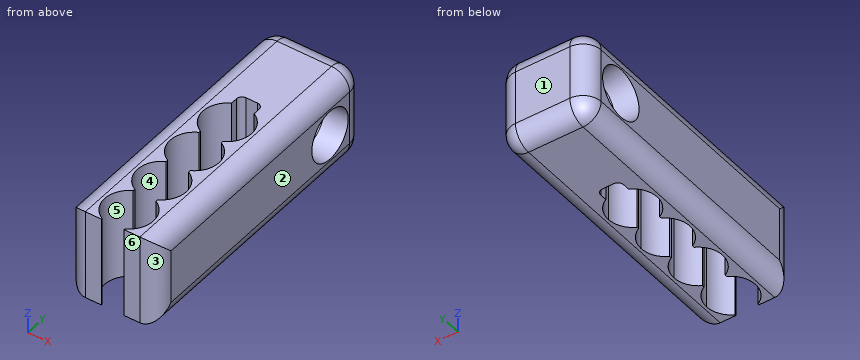
```python
from build123d import *

# Parameters (mm, degrees)
F1_DEPTH = 8
F2_R     = 2.05
F3_DEPTH = 8.001
F4_R     = 1.6
F5_R     = 0.5
F6_SIZE2 = 0.1749773271
F6_SIZE  = 2


with BuildPart() as f1:
    # F0 (on Top) → F1 (new body)
    with BuildSketch(Plane.XY):
        Polygon((1, -4), (4, -4), (4, 4), (-4, 4), (-4, -4), (-1, -4), align=None)
        with BuildLine():
            Line((-1, -5.0967133689), (-1, -4))
            Line((-1, -4), (-4, -4))
            Line((-4, -4), (-4, -21))
            Line((-4, -21), (-1, -21))
            Line((-1, -21), (-1, -20.9032866311))
            ThreePointArc((-1, -20.9032866311), (-2.15, -19), (-1, -17.0967133689))
            Line((-1, -17.0967133689), (-1, -16.9032866311))
            ThreePointArc((-1, -16.9032866311), (-2.15, -15), (-1, -13.0967133689))
            Line((-1, -13.0967133689), (-1, -12.9032866311))
            ThreePointArc((-1, -12.9032866311), (-2.15, -11), (-1, -9.0967133689))
            Line((-1, -9.0967133689), (-1, -8.9032866311))
            ThreePointArc((-1, -8.9032866311), (-2.15, -7), (-1, -5.0967133689))
        make_face()
        with BuildLine():
            Line((4, -21), (4, -4))
            Line((4, -4), (1, -4))
            Line((1, -4), (1, -5.0967133689))
            ThreePointArc((1, -5.0967133689), (1.840176622, -5.8881322021), (2.15, -7))
            ThreePointArc((2.15, -7), (1.840176622, -8.1118677979), (1, -8.9032866311))
            Line((1, -8.9032866311), (1, -9.0967133689))
            ThreePointArc((1, -9.0967133689), (1.840176622, -9.8881322021), (2.15, -11))
            ThreePointArc((2.15, -11), (1.840176622, -12.1118677979), (1, -12.9032866311))
            Line((1, -12.9032866311), (1, -13.0967133689))
            ThreePointArc((1, -13.0967133689), (1.840176622, -13.8881322021), (2.15, -15))
            ThreePointArc((2.15, -15), (1.840176622, -16.1118677979), (1, -16.9032866311))
            Line((1, -16.9032866311), (1, -17.0967133689))
            ThreePointArc((1, -17.0967133689), (1.840176622, -17.8881322021), (2.15, -19))
            ThreePointArc((2.15, -19), (1.840176622, -20.1118677979), (1, -20.9032866311))
            Line((1, -20.9032866311), (1, -21))
            Line((1, -21), (4, -21))
        make_face()
    extrude(amount=F1_DEPTH)

    # F2 (on face) → F3 (cut, through all)
    with BuildSketch(Plane(origin=(-4, 0, 0), x_dir=(0, -1, 0), z_dir=(-1, 0, 0))):
        with Locations((0, 4)):
            Circle(F2_R)
    extrude(amount=-F3_DEPTH, mode=Mode.SUBTRACT)

    # F4
    f4_edges = [f1.edges().sort_by_distance(p)[0] for p in [
        (4, -8.5, 8),
        (4, -8.5, 0),
        (4, 4, 4),
        (4, -21, 4),
        (-4, -21, 4),
        (-4, -8.5, 8),
        (-4, -8.5, 0),
        (-4, 4, 4),
        (0, 4, 8),
        (0, 4, 0),
    ]]
    fillet(f4_edges, radius=F4_R)

    # F5
    f5_edges = [f1.edges().sort_by_distance(p)[0] for p in [
        (1, -4, 4),
        (-1, -4, 4),
    ]]
    fillet(f5_edges, radius=F5_R)

    # F6
    f6_edges = [f1.edges().sort_by_distance(p)[0] for p in [
        (-4, 2.05, 4),
        (4, 2.05, 4),
    ]]
    f6_side = f1.faces().sort_by_distance((0, 2.05, 4))[0]
    chamfer(f6_edges, length=F6_SIZE, length2=F6_SIZE2, reference=f6_side)


solid = f1.part
```
Can you work these out from the model? Positions are in its coordinate system, mm. Face numbers are marked on the shaded views. A direction names the side the tool comes from. Coordinates: 2 decimals unless noted, no trailing zeros. Loops run counter-clockwise (first coordinate to the right, second up) from the corner with the lowest first, then second, coordinate; pieces in that order, holes last. Notation, with made-up numbers: M 58.5,48 L 90.5,48 A18 ccw 90.5,82 Z; hole C 74,63 d10. An arc over 180 degrees is marked long. Put each result on its own line as item: value. Start each with the question number.
(1) Imagine slicing it at C-C on x = -0.25. List the corners of the cut face in (y, z) for me.
(2) Imagine slicing it at B-B on y = 0. List the corners of the cut face in (x, z) for me, and give its area (3 significant figures).
(3) Which directions (+Z, -Z, +X, -X, +Y, -Y) give clear straight access to the entire face, cutting with the end or side of a thin tool? Please do the marked faces 5 and 6.
(4) I need wall thicknesses on probe 1 along Z at (x, y) = (-0.15, 0); probe 2 along X at (y, z) = (-15, 4.25); probe 3 along X at (y, z) = (-13, 2). Which ranges of each line are inside material? Lowest first, please.
(5) Imagine slicing it at A-A on x = 1.5. List the corners of the cut face in (y, z) for me.
(6) We'd pull the mould along Y, two halves only. Please class the marked faces 1, 2, 3 and 4: +Y half, -Y half, draft (parallel to the pull), parting line (faces both ways), or undercut.
Worked answers:
1. outline: M -4,0 L 2.4,0 A1.6 ccw 4,1.6 L 4,6.4 A1.6 ccw 2.4,8 L -4,8 Z; hole C 0,4 d4.1
2. outline: M -4,1.6 A1.6 ccw -2.4,0 L 2.4,0 A1.6 ccw 4,1.6 L 4,1.78 L 2,1.95 L -2,1.95 L -4,1.78 Z; M -4,6.22 L -2,6.05 L 2,6.05 L 4,6.22 L 4,6.4 A1.6 ccw 2.4,8 L -2.4,8 A1.6 ccw -4,6.4 Z
2. area: 28.3 mm2
3. face 5: +Z, -Z
3. face 6: +Z, -Z, +X, -X, -Y
4. probe 1: z = 0 to 1.95, 6.05 to 8
4. probe 2: x = -4 to -2.15, 2.15 to 4
4. probe 3: x = -4 to -1, 1 to 4
5. outline: M -21,0 L -20.54,0 L -20.54,8 L -21,8 Z; M -17.46,0 L -16.54,0 L -16.54,8 L -17.46,8 Z; M -13.46,0 L -12.54,0 L -12.54,8 L -13.46,8 Z; M -9.46,0 L -8.54,0 L -8.54,8 L -9.46,8 Z; M -5.46,0 L 2.4,0 A1.6 ccw 4,1.6 L 4,6.4 A1.6 ccw 2.4,8 L -5.46,8 Z; hole C 0,4 d4.1
6. face 1: +Y half
6. face 2: draft
6. face 3: -Y half
6. face 4: undercut
